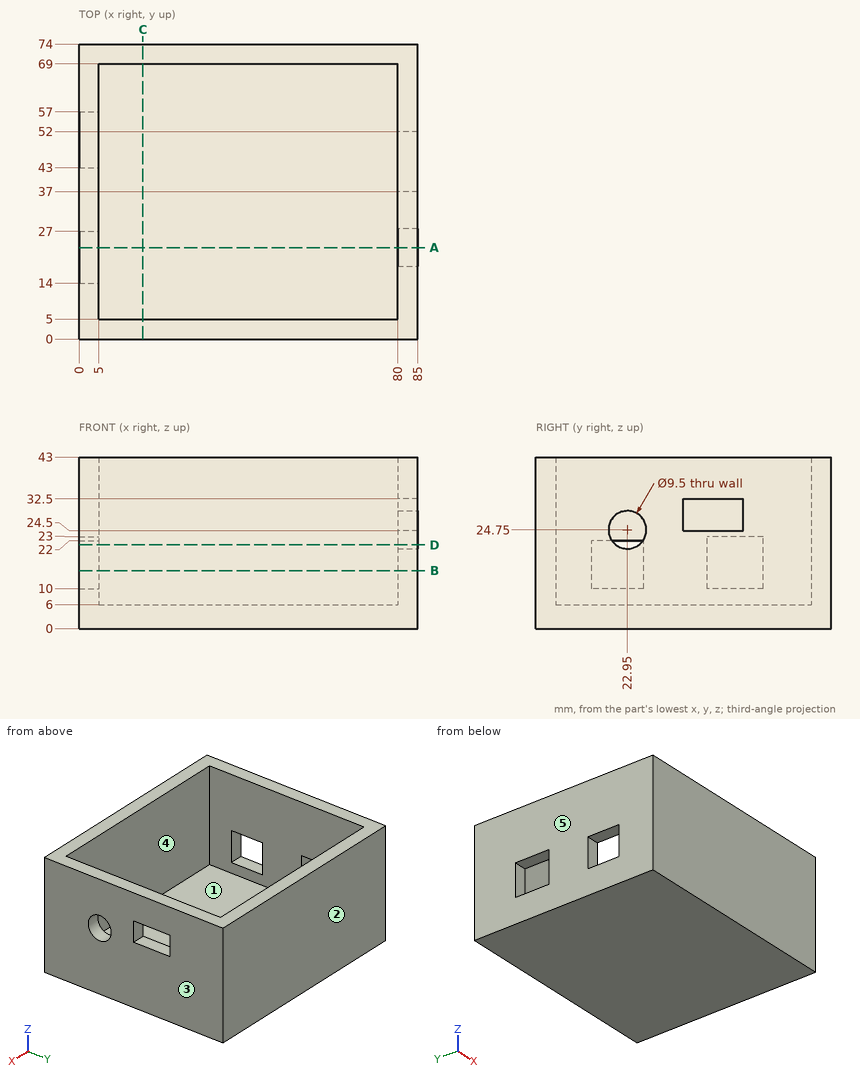
Verification items for this drawing (mm, ordinates from the low corner). A direction names the side the tool comes from. Coordinates: 2 decimals unless noted, no trailing zeros. Order: outer loops, then holes, each group sorted by start corner. A loop starts at its lowest first (then second) coordinate and runs counter-clockwise, first axis right, second up. Notation, with made-up numbers: (-14.5, 62) -> (37.5, 62) arc R17 cw to (37.5, 75) -> close; hole circle Ø11 at (16, 10). An arc over 180 degrees is marked (long way). Put each result on its own line as item: value. Start each with the question number.
1. Access from +Z, -Z, +X, -X, +Y, -Y to the whole of each face (thin tool, end or side, straight path). Record for the marked faces 4 and 5.
2. Cross-section at C-C, the plane x = 16. Record the boundary of the cut face in (y, z).
3. Material ranges on L1, parallel to X at y = 42.5, z = 33.5; L2, parallel to Y at x = 21, z = 14; L3, parallel to Z at x = 81.5, y = 22.95, recorded low to high. Write a range as [from, to].
4. Go/stop test with a flat-tipped pin: pin 1 Ø1 at (x, y) = (48.5, 52.5) entering from +Z. Record where the tip stops, or that it passes through.
5. Cross-section at A-A, the plane y = 22.95. Record the boundary of the cut face in (x, z).
6. Mould release check, pull along X, two halves, no side actions. Record for the marked faces 1, 2 and 3: released by +X, released by -X, zero draft, split by the parting line, or undercut.
7. Cross-section at B-B, the plane z = 14.5. Record the boundary of the cut face in (x, y).
8. Cross-section at D-D, the plane z = 21. Record the boundary of the cut face in (x, y).
Computed:
1. face 4: +Z
1. face 5: +Z, -Z, -X, +Y, -Y
2. outline: (0, 0) -> (74, 0) -> (74, 43) -> (69, 43) -> (69, 6) -> (5, 6) -> (5, 43) -> (0, 43) -> close
3. L1: [0, 5], [80, 85]
3. L2: [0, 5], [69, 74]
3. L3: [0, 20], [29.5, 43]
4. pin 1: z = 6
5. outline: (0, 0) -> (85, 0) -> (85, 20) -> (80, 20) -> (80, 6) -> (5, 6) -> (5, 10) -> (0, 10) -> close; (0, 22) -> (5, 22) -> (5, 43) -> (0, 43) -> close; (80, 29.5) -> (85, 29.5) -> (85, 43) -> (80, 43) -> close
6. face 1: undercut
6. face 2: zero draft
6. face 3: released by +X
7. outline: (0, 0) -> (85, 0) -> (85, 74) -> (0, 74) -> (0, 57) -> (5, 57) -> (5, 69) -> (80, 69) -> (80, 5) -> (5, 5) -> (5, 14) -> (0, 14) -> close; (0, 27) -> (5, 27) -> (5, 43) -> (0, 43) -> close
8. outline: (0, 0) -> (85, 0) -> (85, 20.03) -> (80, 20.03) -> (80, 5) -> (5, 5) -> (5, 14) -> (0, 14) -> close; (0, 27) -> (5, 27) -> (5, 43) -> (0, 43) -> close; (0, 57) -> (5, 57) -> (5, 69) -> (80, 69) -> (80, 25.87) -> (85, 25.87) -> (85, 74) -> (0, 74) -> close
